Could you check a few things on this model? Use its own coordinates, in mm. Give positions to 0.01 mm unless a question says otherwise; leave off trailing zeros. Write each loop counter-clockwise with the first axis right and the second up, starting at its lowest first coordinate (ties: lowest second). Pieces come first, ordered by that corner, then holes. Notation, with made-up numbers: (-5.75, 7.25) -> (44.25, 7.25) arc R24 ccw to (44.25, 18.25) -> close; hole circle Ø4 at (62.25, 67). An arc over 180 degrees is marked (long way). One line per question, with ' | ' between items.
from build123d import *

# Parameters (mm, degrees)
EXTRUDE_1_DEPTH          = 3
EXTRUDE_START            = 2
SKETCH_2_R               = 3
EXTRUDE_2_DEPTH          = 2
SKETCH_3_R               = 3
EXTRUDE_3_DEPTH          = 2
F_3_0_3_DIAMETER_HOLE1_D = 3


with BuildPart() as part:
    # 草图1 → 凸台-拉伸1 (new body)
    with BuildSketch(Plane.XZ):
        with BuildLine():
            ThreePointArc((-6.95625, -2.830629071), (0, -1.645032568), (6.95625, -2.830629071))
            ThreePointArc((6.95625, -2.830629071), (10.95, 0), (6.95625, 2.830629071))
            ThreePointArc((6.95625, 2.830629071), (0, 1.645032568), (-6.95625, 2.830629071))
            ThreePointArc((-6.95625, 2.830629071), (-10.95, 0), (-6.95625, -2.830629071))
        make_face()
    extrude(amount=-EXTRUDE_1_DEPTH)

    # 草图2 → 凸台-拉伸2 (add)
    with BuildSketch(Plane.XZ.offset(EXTRUDE_START)):
        with Locations(Location((7.95, 0, 0), (0, 0, 269.999999998))):
            Circle(SKETCH_2_R)
    extrude(amount=-EXTRUDE_2_DEPTH)

    # 草图3 → 凸台-拉伸3 (add)
    with BuildSketch(Plane.XZ.offset(EXTRUDE_START)):
        with Locations(Location((-7.95, 0, 0), (0, 0, 270))):
            Circle(SKETCH_3_R)
    extrude(amount=-EXTRUDE_3_DEPTH)

    # Ø3.0 (3) Diameter Hole1 (through all)
    with Locations(Plane(origin=(0, 3, 0), x_dir=(1, 0, 0), z_dir=(0, 1, 0))):
        with Locations((-7.95, 0), (7.95, 0)):
            Hole(F_3_0_3_DIAMETER_HOLE1_D / 2)


solid = part.part
Q1. Imagine slicing it at D-D on y = 1.6. Please give me the cut outline in (x, z), and give its area (3 significant figures).
Answer below:
outline: (-6.96, -2.83) arc R21 cw to (6.96, -2.83) arc R3 ccw (long way) to (6.96, 2.83) arc R21 cw to (-6.96, 2.83) arc R3 ccw (long way) to start; hole circle Ø3 at (-7.95, 0); hole circle Ø3 at (7.95, 0) | area: 82.5 mm^2
Q2. Imagine slicing it at C-C on y = -0.8. Please give me the cut outline in (x, z).
Answer below:
outline: circle Ø6 at (-7.95, 0); circle Ø6 at (7.95, 0); hole circle Ø3 at (-7.95, 0); hole circle Ø3 at (7.95, 0)
Q3. Will this pin go through, and if not, where does the flat tip stop? pin 1 (3 mm diameter, centred on x = 2, z = 0.5, fed in from -Y).
Answer below:
pin 1: stops at y = 0
Q4. Imagine slicing it at B-B on x = -7.95. Please give me the cut outline in (y, z).
Answer below:
outline: (-2, -3) -> (3, -3) -> (3, -1.5) -> (-2, -1.5) -> close; (-2, 1.5) -> (3, 1.5) -> (3, 3) -> (-2, 3) -> close
Q5. If I drill on line 1 along Z through (x, y) = (-7.95, 1.65); line 2 along X through (y, z) = (0.9, -1); line 3 along X through (y, z) = (0.3, -1.25), over which ranges is the centre line in solid material (lowest first)?
Answer below:
line 1: z = -3 to -1.5, 1.5 to 3 | line 2: x = -10.78 to -9.07, -6.83 to 6.83, 9.07 to 10.78 | line 3: x = -10.68 to -8.78, -7.12 to 7.12, 8.78 to 10.68
Q6. Imagine slicing it at A-A on z = 0. Please give me the cut outline in (x, y).
Answer below:
outline: (-10.95, -2) -> (-9.45, -2) -> (-9.45, 3) -> (-10.95, 3) -> close; (-6.45, -2) -> (-4.95, -2) -> (-4.95, 0) -> (4.95, 0) -> (4.95, -2) -> (6.45, -2) -> (6.45, 3) -> (-6.45, 3) -> close; (9.45, -2) -> (10.95, -2) -> (10.95, 3) -> (9.45, 3) -> close
Q7. If we mould it in two halves opening along Z, with no side actions, what happens to faces 1 (the cylindrical face through (0.099, 1.479, 1.645)), 2 (the cylindrical face through (6.52, 0.46, -0.45)), 3 (the flat face through (-9.2, -2, -1.3)), 4 (the cylindrical face through (-6.45, 0.46, -0.07))? For each: +Z half, -Z half, draft (parallel to the pull), parting line (faces both ways), or undercut.
Answer below:
face 1: +Z half | face 2: undercut | face 3: draft | face 4: undercut
